Input: part model. Units: mm. Frame: model coordinates. A direction names the side the tool comes from. Give positions to 0.01 mm unless a question says otherwise; leave off trailing zeros. Loops run counter-clockwise (first coordinate to the right, second up) from the corner with the lowest first, then second, coordinate; pieces in that order, holes last. Notation, with made-up numbers: (-4, -3.5) - (14, -3.5) arc R21 cw to (14, 1.5) - close; hole circle Ø6 at (41, 48). An arc over 180 degrees is marked (long way). One line per item, written item: value.
from build123d import *

# Parameters (mm, degrees)
F2_DEPTH = 3


with BuildPart() as f2:
    # F1 (on Top) → F2 (new body)
    with BuildSketch(Plane.XY):
        with BuildLine():
            ThreePointArc((-12.8, -1.363012), (-10.41988, 1.416668), (-6.91069, 2.454538))
            Line((-6.91069, 2.454538), (73.08931, 2.454538))
            ThreePointArc((73.08931, 2.454538), (79.38931, 8.754538), (73.08931, 15.054538))
            Line((73.08931, 15.054538), (-16.91069, 15.054538))
            ThreePointArc((-16.91069, 15.054538), (-21.302441, 13.235416), (-23.121563, 8.843666))
            ThreePointArc((-23.121563, 8.843666), (-33.882827, -3.534816), (-47.637851, 5.4))
            Line((-47.637851, 5.4), (-44.798864, 6.38864))
            ThreePointArc((-44.798864, 6.38864), (-45.098507, 8.182202), (-45.050926, 10))
            Line((-45.050926, 10), (-56.859772, 14.135399))
            ThreePointArc((-56.859772, 14.135399), (-59.175607, 13.881434), (-60.43165, 11.919306))
            ThreePointArc((-60.43165, 11.919306), (-42.336736, -15.237581), (-12.8, -1.363012))
        make_face()
    extrude(amount=F2_DEPTH)


solid = f2.part
Item 1: Section B-B, the plane x = 47. Output: boundary loops of the cut face in (y, z), and give its area (3 significant figures).
Verdict:
outline: (2.45, 0) - (15.05, 0) - (15.05, 3) - (2.45, 3) - close
area: 37.8 mm^2
Item 2: Pin query (flat end, axial travel): P1, Ø8, axis at x = -21, y = -1.5, coming from the -Z side; P2, Ø1, axis at y = 11.5, z = 2.5, coming from the +X side. Return the tip coordinate at first contact, or that it passes through.
Verdict:
P1: stops at z = 0
P2: stops at x = 78.98
Item 3: Draft query along X for faces 1 (the face through (-33.64, -3.5, 1.48)), 2 (the face through (-42.81, -15.1, 1.48)), 3 (the face through (33, 2.455, 1)), 4 (the face through (79.388, 8.616, 1.479)). Return one class per face: pulls with the +X half, pulls with the -X half, needs draft (parallel to the pull), parting line crosses it, or undercut.
Verdict:
face 1: undercut
face 2: parting line crosses it
face 3: needs draft
face 4: pulls with the +X half
Item 4: Access query for faces 5 (the face through (8, 3, 0)), 6 (the face through (-50.873, 12.039, 1.479)), 7 (the face through (-46.2, 5.9, 1.5)). Directions: +Z, -Z, +X, -X, +Y, -Y. A direction counts if a zero-diameter tool reaches every point of the face in a straight line with its end or side. Return the directions, or none.
Verdict:
face 5: -Z, +X, -X, +Y, -Y
face 6: +Z, -Z, +Y
face 7: +Z, -Z
Item 5: Section C-C, the plane y = -9. Output: boundary loops of the cut face in (x, z).
Verdict:
outline: (-53.13, 0) - (-18.11, 0) - (-18.11, 3) - (-53.13, 3) - close
Item 6: Material intervals for L1, parallel to Y at x = 25, z = 1.3; L2, parallel to X at y = 7, z = 0.25; L3, parallel to X at y = -1, z = 1.45, sorted ascending.
Verdict:
L1: y = 2.45 to 15.05
L2: x = -60.55 to -44.94, -23.26 to 79.14
L3: x = -58.6 to -43.33, -27.92 to -12.62
Item 7: Section A-A, the plane z = 1.75. Output: boundary loops of the cut face in (x, y), and give its area (3 significant figures).
Verdict:
outline: (-60.43, 11.92) arc R25 ccw to (-12.8, -1.36) arc R6.45 cw to (-6.91, 2.45) - (73.09, 2.45) arc R6.3 ccw to (73.09, 15.05) - (-16.91, 15.05) arc R6.21 ccw to (-23.12, 8.84) arc R12.5 cw to (-47.64, 5.4) - (-44.8, 6.39) arc R9.5 cw to (-45.05, 10) - (-56.86, 14.14) arc R2.7 ccw to start
area: 1,990 mm^2
